Can you work these out from the drawing? Everything is in mm from the part's minimum corner. A direction names the side the tool comes from. Round coordinates to 2 decimals unless told otherwise and drop trailing zeros. Order: outer loops, then holes, each group sorted by start corner. A loop starts at its lowest first (then second) coordinate and runs counter-clockwise, first axis right, second up. Notation, with made-up numbers: (-38.75, 35) -> (2.25, 35) arc R9 ccw to (2.25, 52) -> close; hole circle Ø1 at (16, 89). An arc over 180 degrees is marked (long way). One line per item, written item: value.
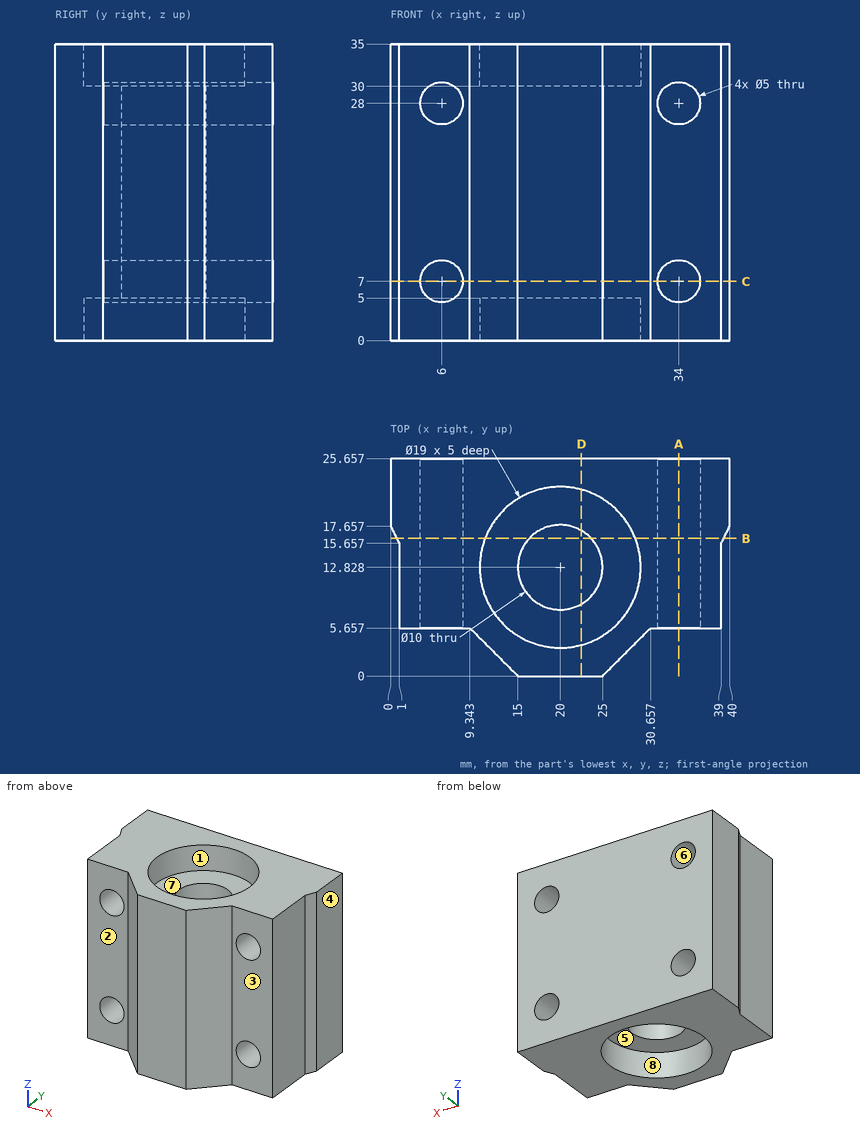
Q1. Will these pins go through, and if not, where does the flat tip stop? pin 1 Ø4 at (y, z) = (14.5, 18) entering from -X; pin 2 Ø4 at (x, z) = (34.5, 19.5) entering from -Y; pin 3 Ø3 at (x, z) = (6, 28) entering from -Y; pin 4 Ø11.5 at (x, y) = (20, 12.83) entering from -Z.
Answers below:
pin 1: x = 0.58
pin 2: y = 5.66
pin 3: through
pin 4: z = 5
Q2. I want a section at C-C on z = 7. List the corners of the cut face in (x, y) for me.
Answers below:
outline: (0, 17.66) -> (1, 15.66) -> (1, 5.66) -> (3.5, 5.66) -> (3.5, 25.66) -> (0, 25.66) -> close; (8.5, 5.66) -> (9.34, 5.66) -> (15, 0) -> (25, 0) -> (30.66, 5.66) -> (31.5, 5.66) -> (31.5, 25.66) -> (8.5, 25.66) -> close; (36.5, 5.66) -> (39, 5.66) -> (39, 15.66) -> (40, 17.66) -> (40, 25.66) -> (36.5, 25.66) -> close; hole circle Ø10 at (20, 12.83)
Q3. I want a section at A-A on x = 34. List the corners of the cut face in (y, z) for me, plus the area to 3 significant figures.
Answers below:
outline: (5.66, 0) -> (25.66, 0) -> (25.66, 4.5) -> (5.66, 4.5) -> close; (5.66, 9.5) -> (25.66, 9.5) -> (25.66, 25.5) -> (5.66, 25.5) -> close; (5.66, 30.5) -> (25.66, 30.5) -> (25.66, 35) -> (5.66, 35) -> close
area: 500 mm^2
Q4. On a 3-axis mill with a long thin cutter (end or side, diameter ignored), from which of +Z, -Z, +X, -X, +Y, -Y can I reach the whole of each face in a straight line? I mean the marked faces 1, 2, 3, 4 and 5. Say none if no direction works.
Answers below:
face 1: +Z
face 2: +Z, -Z, -X, -Y
face 3: +Z, -Z, +X, -Y
face 4: +Z, -Z, +X, +Y, -Y
face 5: -Z
Q5. I want a section at D-D on x = 22.5. List the corners of the cut face in (y, z) for me.
Answers below:
outline: (0, 0) -> (3.66, 0) -> (3.66, 5) -> (8.5, 5) -> (8.5, 30) -> (3.66, 30) -> (3.66, 35) -> (0, 35) -> close; (17.16, 5) -> (21.99, 5) -> (21.99, 0) -> (25.66, 0) -> (25.66, 35) -> (21.99, 35) -> (21.99, 30) -> (17.16, 30) -> close
Q6. We'd pull the mould along Z, two halves only. Please class the marked faces 6, 7 and 8: released by +Z, released by -Z, zero draft, split by the parting line, or undercut.
Answers below:
face 6: undercut
face 7: released by +Z
face 8: zero draft
Q7. I want a section at B-B on y = 16.25. List the corners of the cut face in (x, z) for me.
Answers below:
outline: (0.7, 0) -> (11.14, 0) -> (11.14, 5) -> (16.35, 5) -> (16.35, 30) -> (11.14, 30) -> (11.14, 35) -> (0.7, 35) -> close; (23.65, 5) -> (28.86, 5) -> (28.86, 0) -> (39.3, 0) -> (39.3, 35) -> (28.86, 35) -> (28.86, 30) -> (23.65, 30) -> close; hole circle Ø5 at (6, 7); hole circle Ø5 at (6, 28); hole circle Ø5 at (34, 7); hole circle Ø5 at (34, 28)
Q8. Please list where these lines run through material, in increasing order: line 1 along Z through (x, y) = (34, 11); line 2 along Y through (x, z) = (20, 10.25); line 3 along X through (y, z) = (23, 9).
Answers below:
line 1: 0 to 4.5, 9.5 to 25.5, 30.5 to 35
line 2: 0 to 7.83, 17.83 to 25.66
line 3: 0 to 4.5, 7.5 to 32.5, 35.5 to 40
